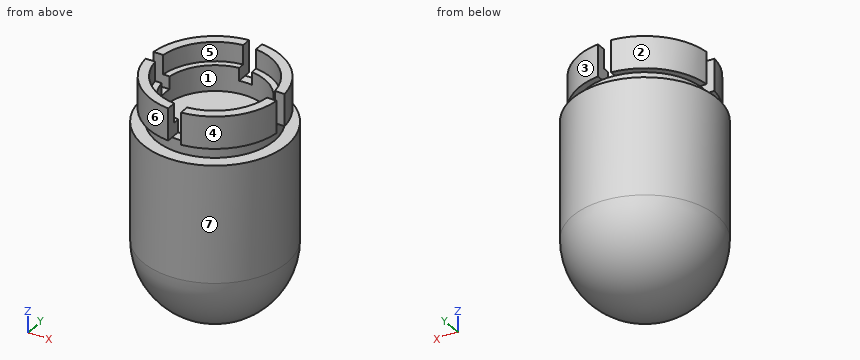
from build123d import *

# Parameters (mm, degrees)
F3_DEPTH      = 25
F3_DEPTH_BACK = 25
F5_DEPTH      = 25
F5_DEPTH_BACK = 25


with BuildPart() as f2:
    # F2: sweep along a path in F1
    with BuildLine(Plane.XY) as f2_path:
        CenterArc((0, 0), 11.25, 0, 360)
    # F0 (on Front) → F2 (sweep)
    with BuildSketch(Plane.XZ):
        with BuildLine():
            Line((10.25, -0.5), (9.25, -0.5))
            Line((9.25, -0.5), (7.75, -0.5))
            Line((7.75, -0.5), (1, -0.5))
            Line((1, -0.5), (0, -0.5))
            Line((0, -0.5), (0, -30))
            ThreePointArc((0, -30), (7.9549512883, -26.7049512883), (11.25, -18.75))
            Line((11.25, -18.75), (11.25, -0.5))
            Line((11.25, -0.5), (10.25, -0.5))
        make_face()
        Polygon((9.25, 1.5), (10.25, 1.5), (10.25, 6.5), (8.75, 6.5), (8.75, 3.5), (7.75, 3.5), (7.75, -0.5), (9.25, -0.5), align=None)
    sweep(path=f2_path.line)

    # F0 (on Front) → F3 (cut, two sides)
    with BuildSketch(Plane.XZ) as f3_sk:
        Polygon((-1, 1.5), (1, 1.5), (1, 6.5), (0, 6.5), (-1, 6.5), align=None)
    extrude(amount=-F3_DEPTH, mode=Mode.SUBTRACT)
    extrude(f3_sk.sketch, amount=F3_DEPTH_BACK, mode=Mode.SUBTRACT)

    # F4 (on Right) → F5 (cut, two sides)
    with BuildSketch(Plane.YZ) as f5_sk:
        Polygon((-1, 1.5), (0, 1.5), (1, 1.5), (1, 6.5), (-1, 6.5), align=None)
    extrude(amount=-F5_DEPTH, mode=Mode.SUBTRACT)
    extrude(f5_sk.sketch, amount=F5_DEPTH_BACK, mode=Mode.SUBTRACT)


solid = f2.part
Here's how the part is built. I have some questions about the finished solid (model axes, mm). Face numbers are marked on the shaded views. A direction names the side the tool comes from. Give positions to 0.01 mm unless a question says otherwise; leave off trailing zeros. Write each loop counter-clockwise with the first axis right and the second up, starting at its lowest first coordinate (ties: lowest second). Pieces come first, ordered by that corner, then holes. Notation, with made-up numbers: (20, 26) -> (29, 26) arc R22 ccw to (29, 60) -> close; hole circle Ø8 at (-2, 15). An arc over 180 degrees is marked (long way). Use one line per item in the form item = value. Start each with the question number.
1. If I drill on L1, parallel to Y at x = 0, z = 0.3; L2, parallel to Y at x = -4.25, z = 5; L3, parallel to Z at x = 2.5, y = 9.5, over which ranges is the centre line in solid material (lowest first)?
2. On a 3-axis mill with a long thin cutter (end or side, diameter ignored), from which of +Z, -Z, +X, -X, +Y, -Y can I reach the whole of each face in a straight line? I mean the marked faces 1, 2, 3 and 4. Say none if no direction works.
3. Thinking about a two-plate mould opening in Y: for the marked faces 5, 6 and 7, which applies, +Y half, -Y half, draft (parallel to the pull), parting line (faces both ways), or undercut?
4. Will these pins go through, and if not, where does the flat tip stop? pin 1 Ø6 at (x, z) = (-8.5, -6.5) entering from -Y; pin 2 Ø6 at (x, z) = (-1, -24) entering from -Y; pin 3 Ø0.8 at (y, z) = (-9.5, 4) entering from -X; pin 4 Ø6 at (y, z) = (-0.5, -6) entering from -X.
5. Imagine slicing it at A-A on z = -3. List the corners of the cut face in (x, y) for me, plus the area to 3 significant figures.
Entries:
q1.L1 = -9.25 to -7.75, 7.75 to 9.25
q1.L2 = -9.33 to -7.65, 7.65 to 9.33
q1.L3 = -24.23 to -0.5, 1.5 to 6.5
q2.face_1 = +Z
q2.face_2 = +Z, -X, +Y
q2.face_3 = +Z, +X, +Y
q2.face_4 = +Z, +X, -Y
q3.face_5 = undercut
q3.face_6 = -Y half
q3.face_7 = parting line
q4.pin_1 = -9.81
q4.pin_2 = -11
q4.pin_3 = -4.72
q4.pin_4 = -11.25
q5.outline = circle Ø22.5 at (0, 0)
q5.area = 398 mm²
